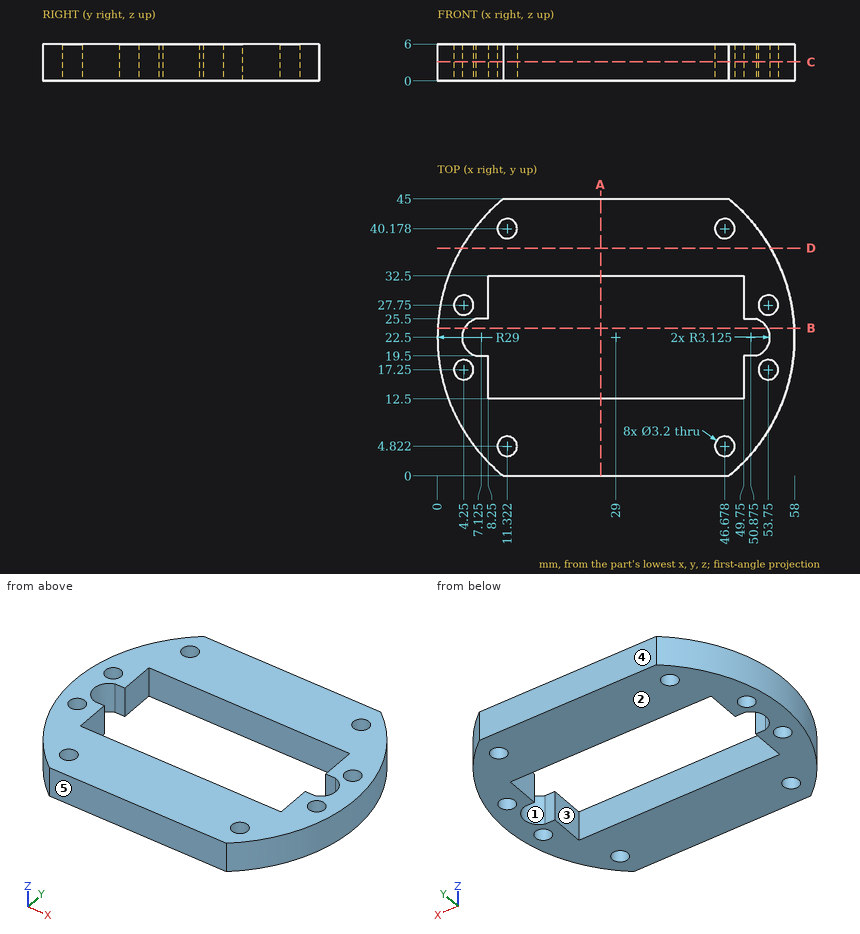
Check sheet for the drawn part. Datum: minimum x, y, z corner. Units: mm. A direction names the side the tool comes from. Round coordinates to 2 decimals unless told otherwise and drop trailing zeros. Order: outer loops, then holes, each group sorted by start corner. A loop starts at its lowest first (then second) coordinate and runs counter-clockwise, first axis right, second up. Notation, with made-up numbers: (38.25, 34.25) -> (59.25, 34.25) arc R16 cw to (59.25, 56.25) -> close; hole circle Ø5 at (32.5, 20). An arc over 180 degrees is marked (long way). Return JSON: item names as keys, results as strings. Group by question number.
Q1. Gauge pin test, flat ends, axial feed: pin 1 (1 mm diameter, centred on y = 16, z = 1.5, fed in from -X); pin 2 (1 mm diameter, centred on y = 20, z = 3, fed in from -X); pin 3 (5 mm diameter, centred on x = 46.68, y = 40.18, fed in from -Z); pin 4 (2.5 mm diameter, centred on x = 53.75, y = 27.75, fed in from -Z). Record the tip position at first contact, or that the pin passes through.
Q2. Release check for a two-part mould opening along Y. For the marked faces 3, 4 and 5 record: released by +Y, released by -Y, zero draft, split by the parting line, or undercut.
Q3. Tool access check on the marked faces 1 and 2. Record the directions out of +Z, -Z, +X, -X, +Y, -Y that give a thin tool (end or side, any length) a straight path to the whole face; none if there is none.
Q4. Section check D-D, the plane y = 37. Record the boundary of the cut face in (x, z) (1 decimal).
Q5. Section check B-B, the plane y = 24. Record the boundary of the cut face in (x, z).
Q6. Section check C-C, the plane z = 3.1. Count the separate pieces of the cut face and the enclosed holes in it, plus the area to 3 significant figures.
Q7. Section check A-A, the plane x = 26.5. Record the boundary of the cut face in (y, z), plus the area to 3 significant figures.
Q8. Material ranges on probe 1 along X at (y, z) = (16.5, 1.4); probe 2 along Y at (x, z) = (22.5, 2.4); probe 3 along X at (y, z) = (27, 5.05), recorded low to high. Write a range as from..to.
Numbers:
{
 "1": {"pin 1": "x = 0.63", "pin 2": "x = 0.07", "pin 3": "z = 0", "pin 4": "through"},
 "2": {"face 3": "undercut", "face 4": "released by +Y", "face 5": "released by -Y"},
 "3": {"face 1": "+Z, -Z", "face 2": "-Z, +X, -X, +Y, -Y"},
 "4": {"outline": "(3.9, 0) -> (54.1, 0) -> (54.1, 6) -> (3.9, 6) -> close"},
 "5": {"outline": "(0.04, 0) -> (4.38, 0) -> (4.38, 6) -> (0.04, 6) -> close; (53.62, 0) -> (57.96, 0) -> (57.96, 6) -> (53.62, 6) -> close"},
 "6": {"separate pieces": "1", "enclosed holes": "9", "area": "1,380 mm^2"},
 "7": {"outline": "(0, 0) -> (12.5, 0) -> (12.5, 6) -> (0, 6) -> close; (32.5, 0) -> (45, 0) -> (45, 6) -> (32.5, 6) -> close", "area": "150 mm^2"},
 "8": {"probe 1": "0.63..2.84, 5.66..8.25, 49.75..52.34, 55.16..57.37", "probe 2": "0..12.5, 32.5..45", "probe 3": "0.35..2.84, 5.66..8.25, 49.75..52.34, 55.16..57.65"}
}
